Geometry check sheet. Reference: the model listing, model coordinates, mm. A direction names the side the tool comes from. Give positions to 0.01 mm unless a question says otherwise; leave off trailing zeros. Write each loop counter-clockwise with the first axis right and the second up, starting at its lowest first coordinate (ties: lowest second). Pieces come first, ordered by that corner, then holes. Notation, with made-up numbers: (2, -8) -> (51, -8) arc R17 cw to (51, 3) -> close; hole circle Ø10 at (62, 31.25). An arc over 180 degrees is marked (long way). One line per item, written item: value.
from build123d import *

# Parameters (mm, degrees)
F0_W          = 134
F0_H          = 80
F1_DEPTH      = 2
F2_W          = 129
F2_H          = 75
F2_W_2        = 123
F2_H_2        = 69
F3_DEPTH      = 2
F3_DEPTH_BACK = 4
F4_W          = 117
F4_H          = 63
F5_DEPTH      = 25


with BuildPart() as f1:
    # F0 (on Top) → F1 (new body)
    with BuildSketch(Plane.XY):
        Rectangle(F0_W, F0_H)
    extrude(amount=F1_DEPTH)

    # F2 (on face) → F3 (join, two sides)
    with BuildSketch(Plane(origin=(0, 0, 0), x_dir=(1, 0, 0), z_dir=(0, 0, -1))) as f3_sk:
        Rectangle(F2_W, F2_H)
        Rectangle(F2_W_2, F2_H_2, mode=Mode.SUBTRACT)
    extrude(amount=F3_DEPTH)
    extrude(f3_sk.sketch, amount=-F3_DEPTH_BACK)

    # F4 (on face) → F5 (cut)
    with BuildSketch(Plane(origin=(0, 0, 0), x_dir=(1, 0, 0), z_dir=(0, 0, -1))):
        Rectangle(F4_W, F4_H)
    extrude(amount=-F5_DEPTH, mode=Mode.SUBTRACT)


solid = f1.part
1) Sectioned sample at A-A on x = 54.5. Record the cut outline in (y, z).
Verdict:
outline: (-40, 0) -> (-37.5, 0) -> (-37.5, -2) -> (-34.5, -2) -> (-34.5, 0) -> (-31.5, 0) -> (-31.5, 2) -> (-34.5, 2) -> (-34.5, 4) -> (-37.5, 4) -> (-37.5, 2) -> (-40, 2) -> close; (31.5, 0) -> (34.5, 0) -> (34.5, -2) -> (37.5, -2) -> (37.5, 0) -> (40, 0) -> (40, 2) -> (37.5, 2) -> (37.5, 4) -> (34.5, 4) -> (34.5, 2) -> (31.5, 2) -> close
2) Tool access check on faces 3 (the flat face through (-5, 36, 4)), 4 (the flat face through (-5, -33, 2)). Record the directions out of +Z, -Z, +X, -X, +Y, -Y that give a thin tool (end or side, any length) a straight path to the whole face; none if there is none.
Verdict:
face 3: +Z, +X, -X, +Y, -Y
face 4: +Z
3) Mould release check, pull along Y, two halves, no side actions. Record for faces 1 (the flat face through (-20, -38, 0)), 2 (the flat face through (-5, -33, 0)): released by +Y, released by -Y, zero draft, split by the parting line, or undercut.
Verdict:
face 1: zero draft
face 2: undercut
4) Sectioned sample at B-B on z = 1.05. Record the cut outline in (x, y), plus the area to 3 significant figures.
Verdict:
outline: (-67, -40) -> (67, -40) -> (67, 40) -> (-67, 40) -> close; hole (-58.5, -31.5) -> (58.5, -31.5) -> (58.5, 31.5) -> (-58.5, 31.5) -> close
area: 3,350 mm^2
5) Scan lines: probe 1 along X at (y, z) = (23, 3); probe 2 along Y at (x, z) = (-13, 1.45); probe 3 along Y at (x, z) = (12, 3.1). Record each from-to range of solid material in increasing order.
Verdict:
probe 1: -64.5 to -61.5, 61.5 to 64.5
probe 2: -40 to -31.5, 31.5 to 40
probe 3: -37.5 to -34.5, 34.5 to 37.5
6) Depth check by flat-ended pin: pin 1 Ø1.6 at (y, z) = (3.5, 3) entering from -X; pin 2 Ø0.6 at (y, z) = (4.5, -1) entering from +X; pin 3 Ø1.6 at (x, z) = (-4, 3) entering from +Y. Enter the tip coordinate at first touch or a pass-through.
Verdict:
pin 1: x = -64.5
pin 2: x = 64.5
pin 3: y = 37.5
7) Sectioned sample at C-C on y = -14. Record the cut outline in (x, z), plus the area to 3 significant figures.
Verdict:
outline: (-67, 0) -> (-64.5, 0) -> (-64.5, -2) -> (-61.5, -2) -> (-61.5, 0) -> (-58.5, 0) -> (-58.5, 2) -> (-61.5, 2) -> (-61.5, 4) -> (-64.5, 4) -> (-64.5, 2) -> (-67, 2) -> close; (58.5, 0) -> (61.5, 0) -> (61.5, -2) -> (64.5, -2) -> (64.5, 0) -> (67, 0) -> (67, 2) -> (64.5, 2) -> (64.5, 4) -> (61.5, 4) -> (61.5, 2) -> (58.5, 2) -> close
area: 58.0 mm^2
